Check sheet for the drawn part. Datum: minimum x, y, z corner. Units: mm. A direction names the side the tool comes from. Give positions to 0.01 mm unless a question says otherwise; leave off trailing zeros. Order: outer loops, then holes, each group sorted by start corner. A loop starts at its lowest first (then second) coordinate and runs counter-clockwise, first axis right, second up.
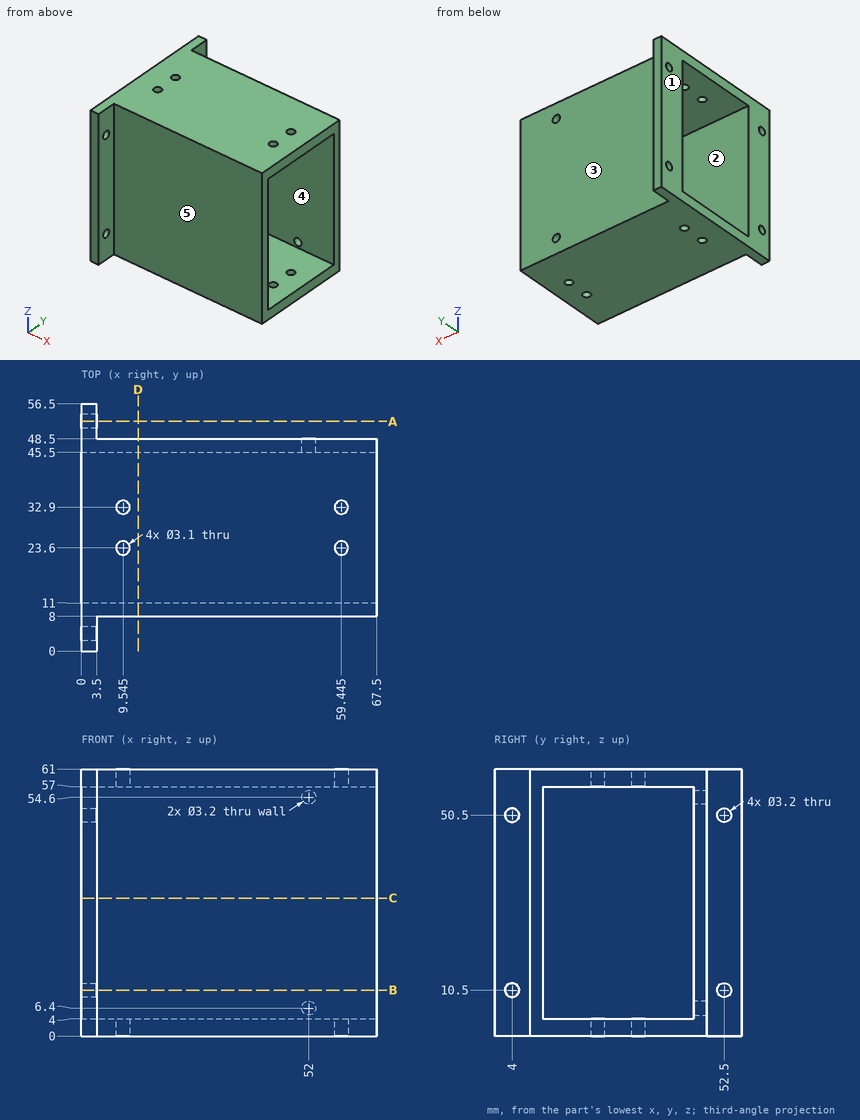
Item 1: Gauge pin test, flat ends, axial feed: pin 1 (4 mm diameter, centred on x = 52, z = 6.4, fed in from -Y); pin 2 (2.5 mm diameter, centred on y = 5, z = 31.5, fed in from +X); pin 3 (5 mm diameter, centred on x = 59.5, z = 12.5, fed in from +Y). Record the tip position at first contact, or that the pin passes through.
Reported:
pin 1: stops at y = 8
pin 2: stops at x = 3.5
pin 3: stops at y = 48.5
Item 2: Sectioned sample at A-A (y = 52.5). Enter the section's corners in (x, z).
Reported:
outline: (0, 0) - (3.5, 0) - (3.5, 8.9) - (0, 8.9) - close; (0, 12.1) - (3.5, 12.1) - (3.5, 48.9) - (0, 48.9) - close; (0, 52.1) - (3.5, 52.1) - (3.5, 61) - (0, 61) - close
Item 3: Scan lines: L1, parallel to Z at x = 2.55, y = 4; L2, parallel to Z at x = 52, y = 47; L3, parallel to Y at x = 17, z = 56. Record each from-to range of solid material in increasing order.
Reported:
L1: z = 0 to 8.9, 12.1 to 48.9, 52.1 to 61
L2: z = 0 to 4.8, 8 to 53, 56.2 to 61
L3: y = 8 to 11, 45.5 to 48.5
Item 4: Sectioned sample at D-D (x = 13). Enter the section's corners in (y, z).
Reported:
outline: (8, 0) - (48.5, 0) - (48.5, 61) - (8, 61) - close; hole (11, 4) - (45.5, 4) - (45.5, 57) - (11, 57) - close
Item 5: Draft check along Y on the marked faces 3, 4 and 5. Enter one of: released by +Y, released by -Y, zero draft, split by the parting line, or undercut.
Reported:
face 3: released by +Y
face 4: undercut
face 5: released by -Y
Item 6: Sectioned sample at B-B (z = 10.5). Enter the section's corners in (x, y).
Reported:
outline: (0, 0) - (3.5, 0) - (3.5, 2.4) - (0, 2.4) - close; (0, 5.6) - (3.5, 5.6) - (3.5, 8) - (67.5, 8) - (67.5, 11) - (0, 11) - close; (0, 45.5) - (67.5, 45.5) - (67.5, 48.5) - (3.5, 48.5) - (3.5, 50.9) - (0, 50.9) - close; (0, 54.1) - (3.5, 54.1) - (3.5, 56.5) - (0, 56.5) - close
Item 7: Set-up check for the marked faces 1 and 2: record each of +Z, -Z, +X, -X, +Y, -Y from which the full face is reachable in a straight line by a thin tool's end or side.
Reported:
face 1: +Z, -Z, -X, +Y, -Y
face 2: +X, -X
Item 8: Sectioned sample at C-C (z = 31.5). Enter the section's corners in (x, y), and give its area (3 significant figures).
Reported:
outline: (0, 0) - (3.5, 0) - (3.5, 8) - (67.5, 8) - (67.5, 11) - (0, 11) - close; (0, 45.5) - (67.5, 45.5) - (67.5, 48.5) - (3.5, 48.5) - (3.5, 56.5) - (0, 56.5) - close
area: 461 mm2
